from build123d import *

# Parameters (mm, degrees)
BOX001_W               = 10
BOX001_H               = 2
BOX001_DEPTH           = 2
BOX001_PLACEMENT_ANGLE = 340
BOX_W                  = 10
BOX_H                  = 2
BOX_DEPTH              = 2
BOX_PLACEMENT_ANGLE    = 20


with BuildPart() as cube001:
    # Box001 → Box001 (new body)
    with BuildSketch(Plane.XY):
        with Locations((5, 1)):
            Rectangle(BOX001_W, BOX001_H)
    extrude(amount=BOX001_DEPTH)


with BuildPart() as cube001_1:
    # Box001 placement: moved
    add(cube001.part.moved(Location((-0.040483, 1.770408, 0))).rotate(Axis((-0.040483, 1.770408, 0), (0, 0, 1)), BOX001_PLACEMENT_ANGLE))


with BuildPart() as fusion:
    # Box → Box (new body)
    with BuildSketch(Plane.XY):
        with Locations((5, 1)):
            Rectangle(BOX_W, BOX_H)
    extrude(amount=BOX_DEPTH)


with BuildPart() as fusion_1:
    # Box placement: moved
    add(fusion.part.moved(Location((0.64, -1.65, 0))).rotate(Axis((0.64, -1.65, 0), (0, 0, 1)), BOX_PLACEMENT_ANGLE))

    # Fusion: union Cube001
    add(cube001_1.part)


solid = fusion_1.part
CAD build for the part. Positions are in the model's coordinates, mm. A direction names the side the tool comes from. Give positions to 0.01 mm unless a question says otherwise; leave off trailing zeros. Loops run counter-clockwise (first coordinate to the right, second up) from the corner with the lowest first, then second, coordinate; pieces in that order, holes last. Notation, with made-up numbers: M -18.5,-40 L 5.5,-40 A30 ccw 5.5,-7 Z; hole C 19,35.5 d2. An arc over 180 degrees is marked long. Answer in a Markdown table with one row per item. Add a question column.
Item 1: Band-saw the part on C-C on x = 0.75. Give the cut face in (y, z).
Item 2: Band-saw the part on D-D on x = 3.25. Give the cut face in (y, z).
Item 3: Probe probe 1 along Y at (x, z) = (9, 1.8); probe 2 along X at (y, z) = (2, 0.5); probe 3 along Y at (x, z) = (4.75, 1.8). List the from-to ranges inside material, lowest first.
Item 4: Band-saw the part on B-B on z = 0.95. Give the cut face in (x, y).
Item 5: Drop flat-ended pins along their axis: P1, Ø1, axis at x = 1.5, z = 1.5, coming from the +Y side; P2, Ø1, axis at x = 5.5, y = 0.5, coming from the -Z side. Give the stop position or say it passes through.
Item 6: Tool access for faces 1 (the face through (1, 1.39, 0.99)), 2 (the face through (2.789, -0.868, 0.986)), 3 (the face through (8.96, 1.38, 0.99)), 4 (the face through (9.7, 2.7, 1)), 5 (the face through (2.79, 2.87, 0.99)): list every direction of +Z, -Z, +X, -X, +Y, -Y with a clear straight run to the whole face (end or side of a thin tool).
Item 7: Mould opens along X. For faces 6 (the face through (9.694, -0.723, 0.986)), 7 (the face through (5, 1, 0)), 8 (the face through (7.145, 2.846, 0.986)) say: +X half, -X half, draft (parallel to the pull), parting line (faces both ways), or undercut.
Item 8: Band-saw the part on A-A on y = 2.5. Give the cut face in (x, z), then the cut area to 3 significant figures.
Reply:
| question | item | result |
|---|---|---|
| 1 | outline | M -1.61,0 L 0.52,0 L 0.52,2 L -1.61,2 Z; M 1.48,0 L 3.61,0 L 3.61,2 L 1.48,2 Z |
| 2 | outline | M -0.7,0 L 2.7,0 L 2.7,2 L -0.7,2 Z |
| 3 | probe 1 | y = -1.52 to 0.61, 1.39 to 3.52 |
| 3 | probe 2 | x = 0.04 to 9.95 |
| 3 | probe 3 | y = -0.15 to 2.16 |
| 4 | outline | M -0.04,0.23 L 0.64,-1.65 L 5,-0.06 L 9.36,-1.65 L 10.04,0.23 L 7.92,1 L 10.04,1.77 L 9.35,3.65 L 5,2.06 L 0.64,3.65 L -0.04,1.77 L 2.07,1 Z |
| 5 | P1 | stops at y = 3.52 |
| 5 | P2 | stops at z = 0 |
| 6 | face 1 | +Z, -Z, -X |
| 6 | face 2 | +Z, -Z, -Y |
| 6 | face 3 | +Z, -Z, +X |
| 6 | face 4 | +Z, -Z, +X, +Y |
| 6 | face 5 | +Z, -Z, +Y |
| 7 | face 6 | +X half |
| 7 | face 7 | draft |
| 7 | face 8 | undercut |
| 8 | outline | M 0.23,0 L 3.8,0 L 3.8,2 L 0.23,2 Z; M 6.19,0 L 9.77,0 L 9.77,2 L 6.19,2 Z |
| 8 | area | 14.3 mm^2 |
